from build123d import *

# Parameters (mm, degrees)
SKETCH2_R           = 2.75
SKETCH2_R_2         = 1.75
BOSS_EXTRUDE1_DEPTH = 2.5
CHAMFER1_SIZE       = 0.25
CHAMFER2_SIZE       = 0.25
CHAMFER3_SIZE       = 0.25
CHAMFER4_SIZE       = 0.25


with BuildPart() as part:
    # Sketch2 → Boss-Extrude1 (new body)
    with BuildSketch(Plane(origin=(0, 0, 0), x_dir=(1, 0, 0), z_dir=(0, 1, 0))):
        Circle(SKETCH2_R)
        Circle(SKETCH2_R_2, mode=Mode.SUBTRACT)
    extrude(amount=BOSS_EXTRUDE1_DEPTH)

    # Chamfer1
    chamfer1_edges = [part.edges().sort_by_distance(p)[0] for p in [
        (-2.75, 2.5, 0),
    ]]
    chamfer(chamfer1_edges, length=CHAMFER1_SIZE)

    # Chamfer2
    chamfer2_edges = [part.edges().sort_by_distance(p)[0] for p in [
        (-2.75, 0, 0),
    ]]
    chamfer(chamfer2_edges, length=CHAMFER2_SIZE)

    # Chamfer3
    chamfer3_edges = [part.edges().sort_by_distance(p)[0] for p in [
        (-1.75, 2.5, 0),
    ]]
    chamfer(chamfer3_edges, length=CHAMFER3_SIZE)

    # Chamfer4
    chamfer4_edges = [part.edges().sort_by_distance(p)[0] for p in [
        (-1.75, 0, 0),
    ]]
    chamfer(chamfer4_edges, length=CHAMFER4_SIZE)


solid = part.part
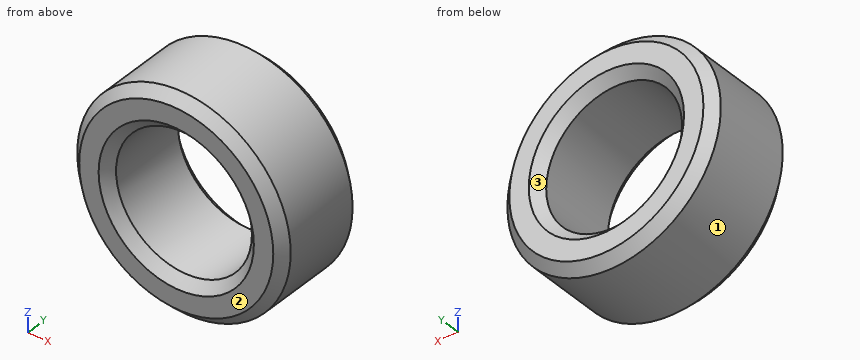
CAD build for the part. Positions are in the model's coordinates, mm. Face numbers are marked on the shaded views. Coordinates: 2 decimals unless noted, no trailing zeros. Loops run counter-clockwise (first coordinate to the right, second up) from the corner with the lowest first, then second, coordinate; pieces in that order, holes last. Notation, with made-up numbers: (4, 38.25) - (44, 38.25) arc R19 cw to (44, 67.25) - close; hole circle Ø11 at (18.5, -22.75). An arc over 180 degrees is marked (long way). Use one line per item in the form item = value. Start each with the question number.
1) Drill centre lines: L1, parallel to Z at x = 0, y = 0.75; L2, parallel to Z at x = -0.05, y = 2.3. Where is each one in solid material? Low to high. Write a range as from..to.
2) Flat gauge pin, fed straight in: pin 1 (1 mm diameter, centred on y = 1, z = -1, fed in from +X). Where does the tip first touch, or does it go through?
3) Band-saw the part on C-C (y = 2.35). Give the cut face in (x, z).
4) Band-saw the part on D-D (y = 1.35). Give the cut face in (x, z), and give its area (3 significant figures).
5) Band-saw the part on A-A (z = 0). Give the cut face in (x, y), and give its area (3 significant figures).
6) Band-saw the part on B-B (x = 0). Give the cut face in (y, z), and give its area (3 significant figures).
7) Two-plate mould, pull along X, no slides. Class the marked faces 1, 2 and 3: +X half, -X half, draft (parallel to the pull), parting line (faces both ways), or undercut.
Check values:
q1.L1 = -2.75..-1.75, 1.75..2.75
q1.L2 = -2.7..-1.8, 1.8..2.7
q2.pin_1 = 2.7
q3.outline = circle Ø5.3 at (0, 0); hole circle Ø3.7 at (0, 0)
q4.outline = circle Ø5.5 at (0, 0); hole circle Ø3.5 at (0, 0)
q4.area = 14.1 mm2
q5.outline = (-2.75, 0.25) - (-2.5, 0) - (-2, 0) - (-1.75, 0.25) - (-1.75, 2.25) - (-2, 2.5) - (-2.5, 2.5) - (-2.75, 2.25) - close; (1.75, 0.25) - (2, 0) - (2.5, 0) - (2.75, 0.25) - (2.75, 2.25) - (2.5, 2.5) - (2, 2.5) - (1.75, 2.25) - close
q5.area = 4.75 mm2
q6.outline = (0, -2.5) - (0.25, -2.75) - (2.25, -2.75) - (2.5, -2.5) - (2.5, -2) - (2.25, -1.75) - (0.25, -1.75) - (0, -2) - close; (0, 2) - (0.25, 1.75) - (2.25, 1.75) - (2.5, 2) - (2.5, 2.5) - (2.25, 2.75) - (0.25, 2.75) - (0, 2.5) - close
q6.area = 4.75 mm2
q7.face_1 = parting line
q7.face_2 = draft
q7.face_3 = undercut
